Geometry: see drawing. Coordinates: mm, zero at the bounding-box minimum. A direction names the side the tool comes from. Coordinates: 2 decimals unless noted, no trailing zeros. Write each loop counter-clockwise with the first axis right and the second up, starting at its lowest first coordinate (ties: lowest second). Pieces come first, ordered by that corner, then holes. Notation, with made-up numbers: M -27.75,65 L -1.75,65 A17 cw -1.75,73 Z; hole C 83.25,-37.5 d3. An arc over 180 degrees is marked long. Write item = value, one per line. Start each with the question number.
1. Line query: line 1 along X through (y, z) = (22, 6); line 2 along X through (y, z) = (31.5, 3); line 3 along Y through (x, z) = (9, 7.5). Output: solid intervals per line, ascending.
2. Section query A-A (y = 48). Output: boundary loops of the cut face in (x, z).
3. Section query D-D (z = 1.5). Output: boundary loops of the cut face in (x, y), then the cut area to 3 significant figures.
4. Pin query (flat end, axial travel): pin 1 Ø3 at (x, y) = (27, 21.5) entering from +Z; pin 2 Ø9 at (x, y) = (15, 26) entering from -Z. Return the tip coordinate at first contact, or that it passes through.
5. Access query for the marked faces 1, 2 and 3. Directions: +Z, -Z, +X, -X, +Y, -Y. A direction counts if a zero-diameter tool reaches every point of the face in a straight line with its end or side. Return the directions, or none.
6. Section query B-B (z = 6.5). Output: boundary loops of the cut face in (x, y).
7. Pull-direction query (X, two-part tool) for the marked faces 4, 5 and 6; classes: pulls with the +X half, pulls with the -X half, needs draft (parallel to the pull), parting line crosses it, or undercut.
8. Section query C-C (x = 26). Output: boundary loops of the cut face in (y, z), then the cut area to 3 significant figures.
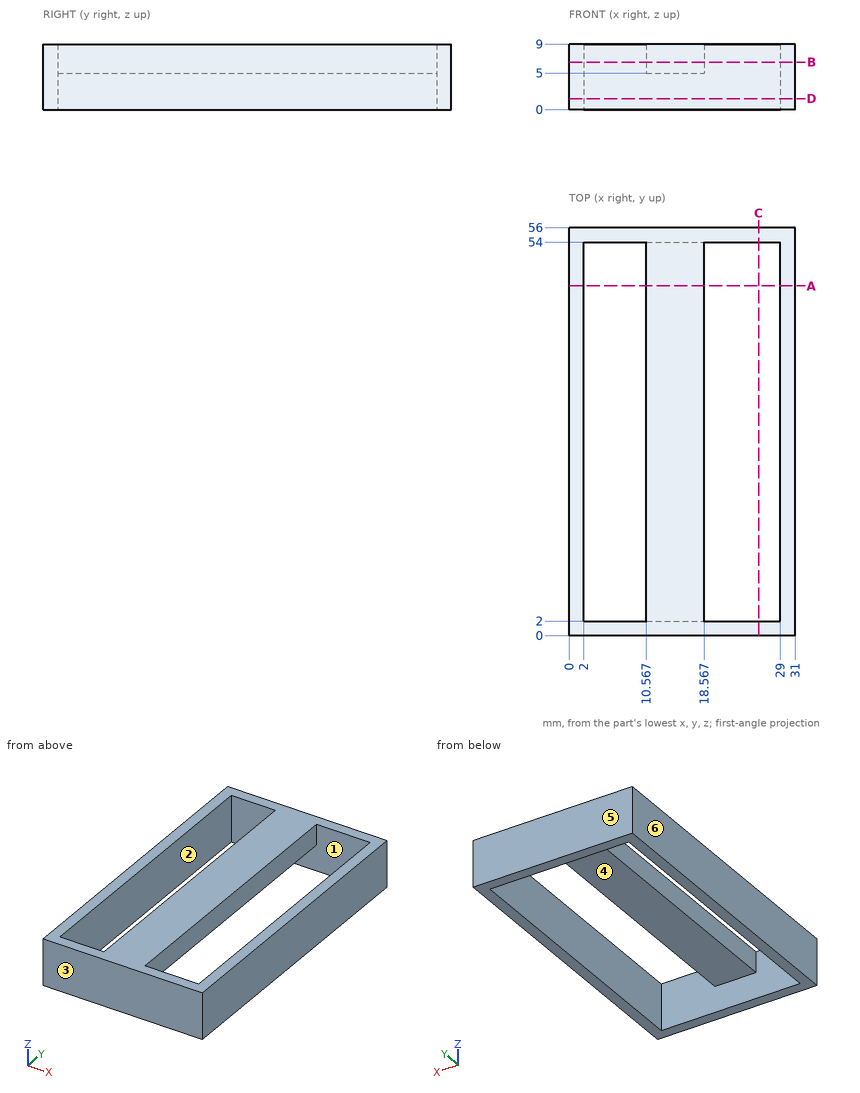
Results are:
q1.line_1 = 0 to 2, 10.57 to 18.57, 29 to 31
q1.line_2 = 0 to 2, 29 to 31
q1.line_3 = 0 to 2, 54 to 56
q2.outline = M 0,0 L 2,0 L 2,9 L 0,9 Z; M 10.57,5 L 18.57,5 L 18.57,9 L 10.57,9 Z; M 29,0 L 31,0 L 31,9 L 29,9 Z
q3.outline = M 0,0 L 31,0 L 31,56 L 0,56 Z; hole M 2,2 L 29,2 L 29,54 L 2,54 Z
q3.area = 332 mm^2
q4.pin_1 = through
q4.pin_2 = 5
q5.face_1 = -Z
q5.face_2 = +Z, -Z
q5.face_3 = +Z, -Z, +X, -X, -Y
q6.outline = M 0,0 L 31,0 L 31,56 L 0,56 Z; hole M 2,2 L 10.57,2 L 10.57,54 L 2,54 Z; hole M 18.57,2 L 29,2 L 29,54 L 18.57,54 Z
q7.face_4 = undercut
q7.face_5 = needs draft
q7.face_6 = pulls with the -X half
q8.outline = M 0,0 L 2,0 L 2,9 L 0,9 Z; M 54,0 L 56,0 L 56,9 L 54,9 Z
q8.area = 36.0 mm^2
